Input: part model. Units: mm. Frame: model coordinates. A direction names the side the tool comes from. Round coordinates to 2 decimals unless told otherwise and drop trailing zeros. Answer as a JSON object with one key per item and string values. Group by question number.
Item 1: Set-up query: faces 1 (the flat face through (150.935, -30, 4)), 2 (the cylindrical face through (56.477, -75.352, 2.465)). Return all of +Z, -Z, +X, -X, +Y, -Y with unobstructed straight access to the full face (end or side cutting, diameter ignored); none if empty.
Item 2: Draft query along X for faces 3 (the flat face through (-149.065, -30, 4)), 4 (the flat face through (-52, -76, 5)), 5 (the flat face through (-1, 122.35, 4)). Return one class per face: released by +X, released by -X, zero draft, split by the parting line, or undercut.
Item 3: Pin query (flat end, axial travel): pin 1 (9.5 mm diameter, centred on x = -49.07, y = -77.65, fed in from -Z); pin 2 (3.5 mm diameter, centred on x = 50.93, y = 22.35, fed in from -Z). Return the tip coordinate at first contact, or that it passes through.
Item 4: Material intervals for line 1 (Y direction, x = -48, z = 6), sorted ascending. Write a range as [from, to].
from build123d import *

# Parameters (mm, degrees)
F0_W     = 300
F0_H     = 300
F1_DEPTH = 9
F2_R     = 3
F3_DEPTH = 9.001
F4_R     = 6
F4_R_2   = 3
F5_DEPTH = 5


with BuildPart() as f1:
    # F0 (on Top) → F1 (new body)
    with BuildSketch(Plane.XY):
        with Locations((0.934564, -27.650428)):
            Rectangle(F0_W, F0_H)
    extrude(amount=F1_DEPTH)

    # F2 (on face) → F3 (cut, through all)
    with BuildSketch(Plane.XY.offset(9)):
        with Locations((-49.065436, 22.349572)):
            Circle(F2_R)
        with Locations((-49.065436, -77.650428)):
            Circle(F2_R)
        with Locations((50.934564, -77.650428)):
            Circle(F2_R)
        with Locations((50.934564, 22.349572)):
            Circle(F2_R)
    extrude(amount=-F3_DEPTH, mode=Mode.SUBTRACT)

    # F4 (on face) → F5 (cut)
    with BuildSketch(Plane(origin=(0, 0, 0), x_dir=(1, 0, 0), z_dir=(0, 0, -1))):
        with Locations((-49.065436, 77.650428)):
            Circle(F4_R)
        with Locations((-49.065436, 77.650428)):
            Circle(F4_R_2, mode=Mode.SUBTRACT)
        with Locations((50.934564, 77.650428)):
            Circle(F4_R)
        with Locations((50.934564, 77.650428)):
            Circle(F4_R_2, mode=Mode.SUBTRACT)
        with Locations((-49.065436, -22.349572)):
            Circle(F4_R)
        with Locations((-49.065436, -22.349572)):
            Circle(F4_R_2, mode=Mode.SUBTRACT)
        with Locations((50.934564, -22.349572)):
            Circle(F4_R)
        with Locations((50.934564, -22.349572)):
            Circle(F4_R_2, mode=Mode.SUBTRACT)
    extrude(amount=-F5_DEPTH, mode=Mode.SUBTRACT)


solid = f1.part
Solved:
{
 "1": {"face 1": "+Z, -Z, +X, +Y, -Y", "face 2": "-Z"},
 "2": {"face 3": "released by -X", "face 4": "undercut", "face 5": "zero draft"},
 "3": {"pin 1": "z = 5", "pin 2": "through"},
 "4": {"line 1": "[-177.65, -80.45], [-74.85, 19.55], [25.15, 122.35]"}
}
